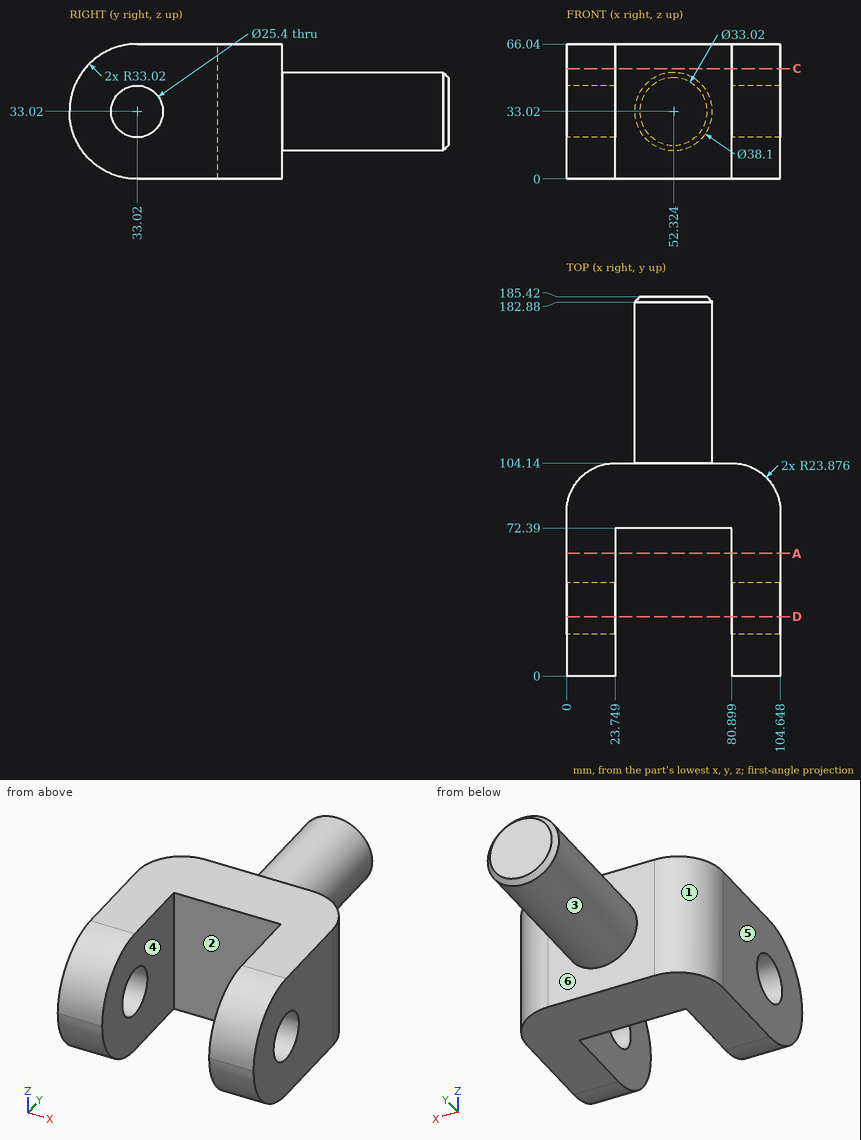
Drawing for the job (mm, zero at the part's lowest x, y, z). A direction names the side the tool comes from. Give positions to 0.01 mm unless a question says otherwise; leave off trailing zeros. Write each loop counter-clockwise with the first axis right and the second up, starting at its lowest first coordinate (ties: lowest second). Pieces come first, ordered by that corner, then holes. Notation, with made-up numbers: M 54.5,14.25 L 99.5,14.25 A21 ccw 99.5,44.25 Z; hole C -7.75,5 d7. An arc over 180 degrees is marked long. Use CSV: the item, a comma, the result in double quotes.
Item 1: Slice it at D-D on y = 29. Write the cut outline in (x, z).
Taken from the geometry:
outline,"M 0,0.25 L 23.75,0.25 L 23.75,20.97 L 0,20.97 Z; M 0,45.07 L 23.75,45.07 L 23.75,65.79 L 0,65.79 Z; M 80.9,0.25 L 104.65,0.25 L 104.65,20.97 L 80.9,20.97 Z; M 80.9,45.07 L 104.65,45.07 L 104.65,65.79 L 80.9,65.79 Z"
Item 2: Pull direction X, two halves, no side cores. Call the marked faces 4, 5 and 6: +X half, -X half, draft (parallel to the pull), parting line (faces both ways), or undercut.
Taken from the geometry:
face 4,"undercut"
face 5,"-X half"
face 6,"draft"
Item 3: Slice it at C-C on z = 54. Write the cut outline in (x, y).
Taken from the geometry:
outline,"M 0,7.52 L 23.75,7.52 L 23.75,72.39 L 80.9,72.39 L 80.9,7.52 L 104.65,7.52 L 104.65,80.26 A23.88 ccw 80.77,104.14 L 23.88,104.14 A23.88 ccw 0,80.26 Z"
Item 4: Which spindle directions (+Z, -Z, +X, -X, +Y, -Y) get a long thin tool onto all of the face, cutting with end or side? Do the marked faces 1, 2 and 3. Say none if no direction does.
Taken from the geometry:
face 1,"+Z, -Z, -X, +Y"
face 2,"+Z, -Z, -Y"
face 3,"+Y"
Item 5: Drill centre lines: probe 1 along X at (y, z) = (50.5, 46); probe 2 along Z at (x, y) = (13, 33); probe 3 along Y at (x, z) = (80.5, 23). Where is each one in solid material? Low to high.
Taken from the geometry:
probe 1,"x = 0 to 23.75, 80.9 to 104.65"
probe 2,"z = 0 to 20.32, 45.72 to 66.04"
probe 3,"y = 72.39 to 104.14"
Item 6: Slice it at A-A on y = 60. Write the cut outline in (x, z), plus the area to 3 significant figures.
Taken from the geometry:
outline,"M 0,0 L 23.75,0 L 23.75,66.04 L 0,66.04 Z; M 80.9,0 L 104.65,0 L 104.65,66.04 L 80.9,66.04 Z"
area,"3,140 mm²"
Item 7: Pin check, flat tips, straight feed: P1, Ø1, axis at x = 13.5, z = 40.5, coming from the -Y side; P2, Ø5, axis at x = 23, z = 23, coming from the +Y side; P3, Ø5, axis at x = 57, y = 154, coming from the +Z side; P4, Ø8, axis at x = 27, y = 136, coming from the +Z side. Stop position of each tip, or through.
Taken from the geometry:
P1,"stops at y = 0.75"
P2,"stops at y = 104.14"
P3,"stops at z = 51.95"
P4,"passes through"
